Geometry: final body of the model. Coordinates: model frame, mm. Give positions to 0.01 mm unless a question says otherwise; leave off trailing zeros. Write each loop counter-clockwise with the first axis right and the second up, starting at its lowest first coordinate (ties: lowest second). Pieces come first, ordered by that corner, then holes. Notation, with made-up numbers: M -11,-11.75 L 9,-11.75 A29 ccw 9,24.25 Z; hole C 80.25,-23.5 d6. An arc over 180 degrees is marked long. Answer as a JSON object with one key per item and string values.
from build123d import *

# Parameters (mm, degrees)
SKETCH_1_R      = 0.6
SKETCH_1_R_2    = 0.2
EXTRUDE_1_DEPTH = 0.2
EXTRUDE_START   = -0.2
EXTRUDE_2_DEPTH = 0.2
FILLET_1_R      = 0.2
FILLET_2_R      = 0.05


with BuildPart() as part:
    # Эскиз1 → Бобышка-Вытянуть1 (new body)
    with BuildSketch(Plane.XY):
        Circle(SKETCH_1_R)
        Circle(SKETCH_1_R_2, mode=Mode.SUBTRACT)
    extrude(amount=EXTRUDE_1_DEPTH)

    # Эскиз3 → Бобышка-Вытянуть2 (add)
    with BuildSketch(Plane.XY.offset(0.2).offset(EXTRUDE_START)):
        with BuildLine():
            Line((-0.2, 0.565685425), (-0.2, 14))
            Line((-0.2, 14), (0.2, 14))
            Line((0.2, 14), (0.2, 0.565685425))
            ThreePointArc((0.2, 0.565685425), (0, 0.6), (-0.2, 0.565685425))
        make_face()
        with BuildLine():
            Line((-0.2, -0.565685425), (-0.473607186, -1.89863889))
            ThreePointArc((-0.473607186, -1.89863889), (-0.53485247, -2.514130031), (-0.468572045, -3.129099328))
            Line((-0.468572045, -3.129099328), (-0.4, -3.44981817))
            Line((-0.4, -3.44981817), (0.4, -3.44981817))
            Line((0.4, -3.44981817), (0.468572045, -3.129099328))
            ThreePointArc((0.468572045, -3.129099328), (0.53485247, -2.514130031), (0.473607186, -1.89863889))
            Line((0.473607186, -1.89863889), (0.2, -0.565685425))
            ThreePointArc((0.2, -0.565685425), (0, -0.6), (-0.2, -0.565685425))
        make_face()
    extrude(amount=EXTRUDE_2_DEPTH)

    # Скругление1
    fillet_1_edges = [part.edges().sort_by_distance(p)[0] for p in [
        (-0.4, -3.44981817, 0.1),
        (0.4, -3.44981817, 0.1),
        (-0.2, 14, 0.1),
        (0.2, 14, 0.1),
    ]]
    fillet(fillet_1_edges, radius=FILLET_1_R - 0.0001)  # a hair under: the kernel refuses the full size

    # Скругление2
    fillet_2_edges = [part.edges().sort_by_distance(p)[0] for p in [
        (0.2, 7.182892712, 0.2),
        (0.6, 0, 0.2),
        (-0.336803593, -1.232162158, 0.2),
        (-0.53485247, -2.514130031, 0.2),
        (-0.451187979, -3.210406476, 0.2),
        (0.53485247, -2.514130031, 0.2),
        (0.336803593, -1.232162158, 0.2),
        (0, -3.44981817, 0.2),
        (0.451187979, -3.210406476, 0.2),
        (-0.2, 7.182892712, 0.2),
        (0.364030264, -3.405344875, 0.2),
        (-0.364030264, -3.405344875, 0.2),
        (0.141450646, 13.941450646, 0.2),
        (-0.141450646, 13.941450646, 0.2),
        (-0.2, 0, 0.2),
        (-0.6, 0, 0.2),
    ]]
    fillet(fillet_2_edges, radius=FILLET_2_R)


solid = part.part
1) Cut plane C-C on y = 3. Return loops of the section in (x, z), and give its area (3 significant figures).
Geometry check:
{"outline": "M -0.2,0 L 0.2,0 L 0.2,0.15 A0.05 ccw 0.15,0.2 L -0.15,0.2 A0.05 ccw -0.2,0.15 Z", "area": "0.0789 mm2"}
2) Line query: line 1 (Y direction, x = 0, z = 0.1); line 2 (X direction, y = 3, z = 0.1); line 3 (X direction, y = -0.5, z = 0.1). Output: solid intervals per line, ascending. Write a range as from..to.
Geometry check:
{"line 1": "y = -3.45..-0.2, 0.2..14", "line 2": "x = -0.2..0.2", "line 3": "x = -0.33..0.33"}
3) Cut plane B-B on y = 0. Return loops of the section in (x, z), and give its area (3 significant figures).
Geometry check:
{"outline": "M -0.6,0 L -0.2,0 L -0.2,0.15 A0.05 ccw -0.25,0.2 L -0.55,0.2 A0.05 ccw -0.6,0.15 Z; M 0.2,0 L 0.6,0 L 0.6,0.15 A0.05 ccw 0.55,0.2 L 0.25,0.2 A0.05 ccw 0.2,0.15 Z", "area": "0.158 mm2"}
